Build history of the part. All positions in model axes, mm. A direction names the side the tool comes from. Coordinates: 2 decimals unless noted, no trailing zeros. Order: outer loops, then holes, each group sorted by start corner. A loop starts at its lowest first (then second) coordinate and runs counter-clockwise, first axis right, second up. Notation, with made-up numbers: (37, 41) - (46, 41) arc R18 ccw to (46, 72) - close; hole circle Ø10 at (85.5, 87). An arc over 180 degrees is marked (long way). Answer as CSV lines item,"result". Start each with the question number.
from build123d import *

# Parameters (mm, degrees)
CHAMFER1_SIZE = 0.5


with BuildPart() as part:
    # Sketch1 → Revolve1 (revolve)
    with BuildSketch(Plane.XY):
        Polygon((0, 3.96875), (0, 5.96875), (-3, 5.96875), (-3, 0), (31.5366, 0), (31.5366, 3.96875), (30.0366, 3.96875), (30.0366, 3.683), (29.3, 3.683), (29.3, 3.96875), align=None)
    revolve(axis=Axis((-20.199082849, 0, 0), (1, 0, 0)))

    # Chamfer1
    chamfer1_edges = [part.edges().sort_by_distance(p)[0] for p in [
        (0, -3.96875, 0),
        (-3, -5.96875, 0),
        (31.5366, -3.96875, 0),
    ]]
    chamfer(chamfer1_edges, length=CHAMFER1_SIZE)


solid = part.part
(1) Probe L1, parallel to X at y = -1, z = 4.5; L2, parallel to Z at x = 30.5, y = -1.25; L3, parallel to Z at x = 21, y = -3.5. List the from-to ranges inside material, lowest first. Write a range as [from, to].
(2) Pull direction X, two halves, no side cores. Call faces 3 (the cylindrical face through (29.663, 1.699, -3.267)), 4 (the cylindrical face through (30.53, -0.86, -3.874)), 5 (the flat face through (-3, 0, 0)): +X half, -X half, draft (parallel to the pull), parting line (faces both ways), or undercut.
(3) Which spindle directions (+Z, -Z, +X, -X, +Y, -Y) get a long thin tool onto all of the face, cutting with end or side? Do faces 1 (the flat face through (0, -1.3, 4.45)), 2 (the cylindrical face through (-1.268, -1.294, -5.827)). Say none if no direction does.
(4) Drop flat-ended pins along their axis: pin 1 Ø2 at (x, z) = (20, -3.5) entering from -Y; pin 2 Ø6 at (x, y) = (24, -4) entering from -Z; pin 3 Ø5 at (x, z) = (13, 4.5) entering from +Y. Give the stop position or say it passes through.
(5) Band-saw the part on C-C on x = 17. List the corners of the cut face in (y, z).
(6) Band-saw the part on A-A on z = 0. List the corners of the cut face in (x, y).
Filled in:
1,L1,"x = [-3, 0]"
1,L2,"z = [-3.77, 3.77]"
1,L3,"z = [-1.87, 1.87]"
2,face 3,"undercut"
2,face 4,"draft"
2,face 5,"-X half"
3,face 1,"+X"
3,face 2,"+X, -X"
4,pin 1,"stops at y = -3.08"
4,pin 2,"stops at z = -3.84"
4,pin 3,"stops at y = 3.43"
5,outline,"circle Ø7.94 at (0, 0)"
6,outline,"(-3, -5.47) - (-2.5, -5.97) - (0, -5.97) - (0, -4.47) - (0.5, -3.97) - (29.3, -3.97) - (29.3, -3.68) - (30.04, -3.68) - (30.04, -3.97) - (31.04, -3.97) - (31.54, -3.47) - (31.54, 3.47) - (31.04, 3.97) - (30.04, 3.97) - (30.04, 3.68) - (29.3, 3.68) - (29.3, 3.97) - (0.5, 3.97) - (0, 4.47) - (0, 5.97) - (-2.5, 5.97) - (-3, 5.47) - close"
